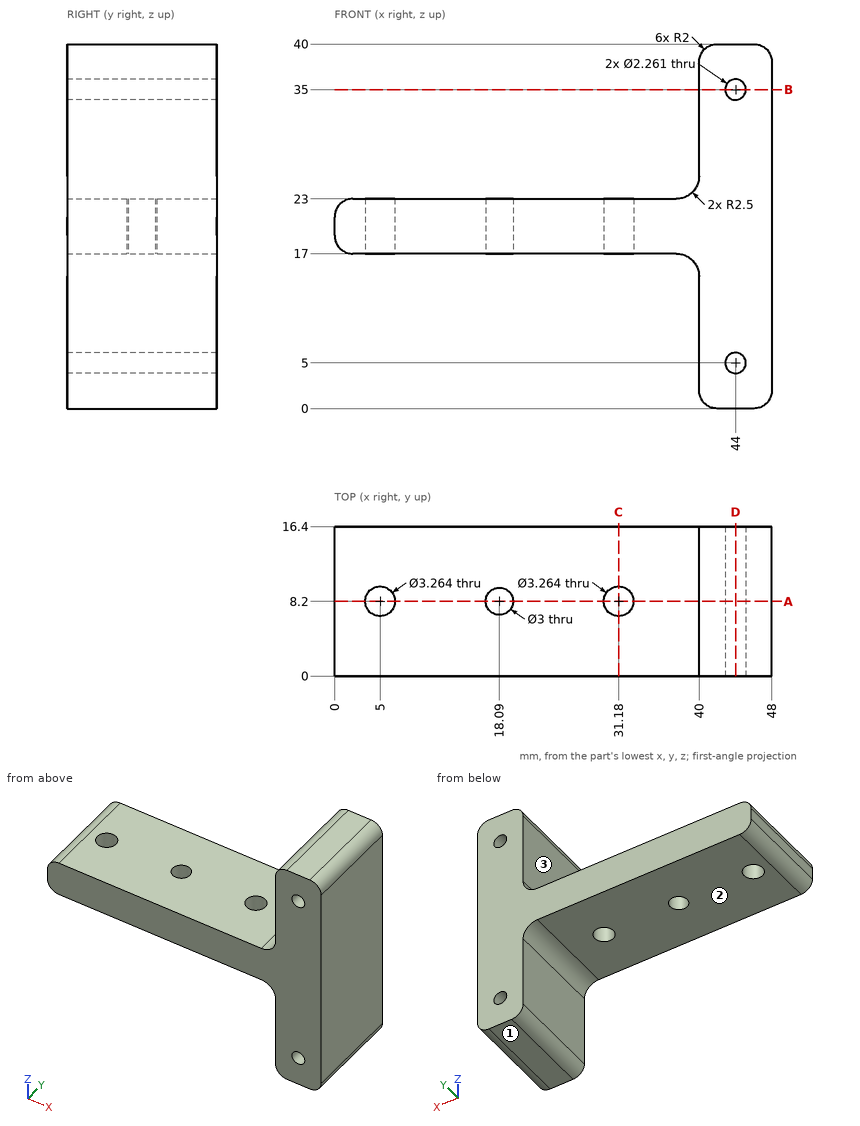
Geometry: see drawing. Coordinates: mm, zero at the bounding-box minimum. A direction names the side the tool comes from. Round coordinates to 2 decimals unless told otherwise and drop trailing zeros. Write each loop counter-clockwise with the first axis right and the second up, starting at its lowest first coordinate (ties: lowest second). Pieces come first, ordered by that corner, then holes. Notation, with made-up numbers: (54, 68) - (103, 68) arc R17 ccw to (103, 90) - close; hole circle Ø3 at (13.5, 8). An arc over 180 degrees is marked (long way). Use CSV: the item, a comma, the result in double quotes. Start each with the question number.
(1) Cut plane D-D, the plane x = 44. Return loops of the section in (y, z).
(2) Cut plane B-B, the plane z = 35. Return loops of the section in (x, y).
(3) Cut plane A-A, the plane y = 8.2. Give the number of separate pieces and of enclosed holes in the cut face, and give its area (3 significant figures).
(4) Set-up query: the marked faces 1, 2 and 3. Return all of +Z, -Z, +X, -X, +Y, -Y with unobstructed straight access to the full face (end or side cutting, diameter ignored); none if empty.
(5) Cut plane C-C, the plane x = 31.18. Return loops of the section in (y, z).
(6) First-contact query: pin 1 Ø8 at (x, y) = (13, 8.5) entering from +Z; pin 2 Ø6 at (y, z) = (5.5, 33) entering from -X; pin 3 Ø2.5 at (x, y) = (18.09, 8.2) entering from -Z; pin 4 Ø5 at (y, z) = (9.5, 26.5) entering from -X. Flat tips, straight axial feed; report the tip coordinate or a pass-through.
(7) Material intervals for probe 1 along Z at (x, y) = (44, 6); probe 2 along Y at (x, z) = (18, 19); probe 3 along Y at (x, z) = (5, 18), sorted ascending. Write a range as [from, to].
Geometry says:
1,outline,"(0, 0) - (16.4, 0) - (16.4, 3.87) - (0, 3.87) - close; (0, 6.13) - (16.4, 6.13) - (16.4, 33.87) - (0, 33.87) - close; (0, 36.13) - (16.4, 36.13) - (16.4, 40) - (0, 40) - close"
2,outline,"(40, 0) - (42.87, 0) - (42.87, 16.4) - (40, 16.4) - close; (45.13, 0) - (48, 0) - (48, 16.4) - (45.13, 16.4) - close"
3,separate pieces,"4"
3,enclosed holes,"2"
3,area,"492 mm²"
4,face 1,"-Z, +X, -X, +Y, -Y"
4,face 2,"-Z, -X, +Y, -Y"
4,face 3,"+Z, -X, +Y, -Y"
5,outline,"(0, 17) - (6.57, 17) - (6.57, 23) - (0, 23) - close; (9.83, 17) - (16.4, 17) - (16.4, 23) - (9.83, 23) - close"
6,pin 1,"z = 23"
6,pin 2,"x = 40"
6,pin 3,"through"
6,pin 4,"x = 39.5"
7,probe 1,"[0, 3.87], [6.13, 33.87], [36.13, 40]"
7,probe 2,"[0, 6.7], [9.7, 16.4]"
7,probe 3,"[0, 6.57], [9.83, 16.4]"
